Could you check a few things on this model? Use its own coordinates, in mm. Give positions to 0.01 mm unless a question says otherwise; leave off trailing zeros. Order: outer loops, then holes, each group sorted by start corner. A loop starts at its lowest first (then second) coordinate and runs counter-clockwise, first axis right, second up.
Autodesk Inventor part; units mm, degrees
ref_plane "YZ Plane" through (0, 0, 0) normal (1, 0, 0) x (0, 1, 0)
ref_plane "XZ Plane" through (0, 0, 0) normal (0, 1, 0) x (-1, 0, 0)
ref_plane "XY Plane" through (0, 0, 0) normal (0, 0, 1) x (1, 0, 0)
sketch "Sketch1" plane through (0, 0, 0) normal (1, 0, 0) x (0, 1, 0)
  line L0 (0, 78.3368) -> (0, 427.0775)
  line L1 (9.8481, 428.814) -> (120.1519, 448.2635)
  line L2 (131.7365, 440.1519) -> (154.2135, 312.6787)
  line L3 (503.1119, 189.3047) -> (590.8645, 150.2346)
  line L4 (595.9326, 137.0318) -> (559.5861, 55.3964)
  line L5 (494.9423, 192.942) -> (494.9423, 192.942)
  line L6 (442.0149, 172.9748) -> (165.6696, 297.928)
  arc A0 (442.0149, 172.9748) -> (490.9347, 186.0198) centre (458.495, 209.4221) ccw
  arc A1 (154.2135, 312.6787) -> (165.6696, 297.928) centre (173.9096, 316.1516) ccw
  arc A2 (131.7365, 440.1519) -> (120.1519, 448.2635) centre (121.8884, 438.4154) ccw
  line L7 (9.8481, 428.814) -> (0, 417.0775)
  arc A3 (595.9326, 137.0318) -> (590.8645, 150.2346) centre (586.7972, 141.0991) ccw
  arc A4 (503.1119, 189.3047) -> (490.9347, 186.0198) centre (499.0446, 180.1692) ccw
  line L8 (9.651, 68.3429) -> (550.1017, 49.4699)
  arc A5 (550.1017, 49.4699) -> (559.5861, 55.3964) centre (550.4507, 59.4638) ccw
  arc A6 (0, 78.3368) -> (9.651, 68.3429) centre (10, 78.3368) ccw
  line L9 (0, 417.0775) -> (0, 78.3368)
  point P0 (534.922, 0)
  point P1 (130, 450)
  point P2 (156.0472, 302.2788)
  point P3 (600, 146.1672)
  point P4 (478.4622, 156.4947)
  point P5 (0, 427.0775)
  point P6 (0, 28.3368)
  dimension "d0" = 130
  dimension "d1" = 404.922
  dimension "d3" = 150
  dimension "d4" = 160
  dimension "d5" = 115
  dimension "d13" = 40
  dimension "d14" = 40
  dimension "d15" = 20
  dimension "d16" = 10
  dimension "d17" = 10
  dimension "d18" = 10
  dimension "d68" = 10
  dimension "d69" = 10
extrude "Extrusion1" add sketch "Sketch1" along normal blind 16
sketch "Sketch2" plane through (16, 0, 0) normal (1, 0, 0) x (0, 0, -1)
  line L0 (-172.9748, 442.0149) -> (-297.928, 165.6696)
  line L1 (-428.814, 9.8481) -> (-417.0775, 0)
  line L2 (-417.0775, 0) -> (-78.3368, 0)
  line L3 (-55.3964, 559.5861) -> (-137.0318, 595.9326)
  arc A0 (-137.0318, 595.9326) -> (-150.2346, 590.8645) centre (-141.0991, 586.7972) ccw
  line L4 (-150.2346, 590.8645) -> (-189.3047, 503.1119)
  arc A1 (-189.3047, 503.1119) -> (-186.0198, 490.9347) centre (-180.1692, 499.0446) ccw
  arc A2 (-172.9748, 442.0149) -> (-186.0198, 490.9347) centre (-209.4221, 458.495) ccw
  line L5 (-172.9748, 442.0149) -> (-297.928, 165.6696)
  arc A3 (-312.6787, 154.2135) -> (-297.928, 165.6696) centre (-316.1516, 173.9096) ccw
  line L6 (-312.6787, 154.2135) -> (-440.1519, 131.7365)
  arc A4 (-440.1519, 131.7365) -> (-448.2635, 120.1519) centre (-438.4154, 121.8884) ccw
  line L7 (-448.2635, 120.1519) -> (-428.814, 9.8481)
  line L8 (-438.4154, 121.8884) -> (-310.9422, 144.3654)
  line L9 (-286.9073, 160.6932) -> (-163.5511, 437.7551)
  line L10 (-163.5511, 437.7551) -> (-143.4328, 482.9414)
  line L11 (-143.4328, 482.9414) -> (-139.4594, 491.8657)
  line L12 (-139.4594, 491.8657) -> (-130.324, 487.7983)
  line L13 (-130.324, 487.7983) -> (-288.9516, 131.5158)
  line L14 (-288.9516, 131.5158) -> (-298.087, 135.5831)
  line L15 (-298.087, 135.5831) -> (-286.9073, 160.6932)
  line L16 (-428.814, 9.8481) -> (-417.0775, 0)
  line L17 (-143.5969, 482.7615) -> (-143.5268, 482.7303)
  line L18 (-438.4154, 121.8884) -> (-303.4968, 145.6782)
  line L19 (-303.4968, 145.6782) -> (-301.7603, 135.8301)
  line L20 (-301.7603, 135.8301) -> (-436.679, 112.0403)
  line L21 (-438.4154, 121.8884) -> (-436.679, 112.0403)
  line L22 (-436.679, 112.0403) -> (-417.404, 2.7267)
  line L23 (-436.679, 112.0403) -> (-325.679, 112.0403) construction
  line L24 (-417.404, 2.7267) -> (-407.5559, 4.4631)
  line L25 (-407.5559, 4.4631) -> (-426.8309, 113.7768)
  line L26 (-141.0991, 586.7972) -> (-182.9931, 492.702)
  line L27 (-182.9931, 492.702) -> (-173.8576, 488.6347)
  line L28 (-173.8576, 488.6347) -> (-131.9637, 582.7298)
  line L29 (-139.4594, 491.8657) -> (-166.9664, 504.1126)
  line L30 (-139.4594, 491.8657) -> (-109.3492, 491.8657) construction
  line L31 (-166.9664, 504.1126) -> (-171.0338, 494.9772)
  line L32 (-171.0338, 494.9772) -> (-143.5268, 482.7303)
  line L33 (-141.0991, 586.7972) -> (-131.9637, 582.7298)
  line L34 (-131.9637, 582.7298) -> (3.0363, 582.7298) construction
  line L35 (-12.7024, 518.6849) -> (487.2976, 518.6849) construction
  line L36 (-288.9516, 131.5158) -> (-274.7158, 163.4898)
  line L37 (-274.7158, 163.4898) -> (-214.4218, 136.6452)
  line L38 (-214.4218, 136.6452) -> (-218.4892, 127.5097)
  line L39 (-218.4892, 127.5097) -> (-278.7831, 154.3544)
  line L40 (-68.3429, 9.651) -> (-49.4699, 550.1017)
  arc A5 (-49.4699, 550.1017) -> (-55.3964, 559.5861) centre (-59.4638, 550.4507) ccw
  arc A6 (-78.3368, 0) -> (-68.3429, 9.651) centre (-78.3368, 10) ccw
  line L41 (-131.9637, 582.7298) -> (-54.3123, 548.1572)
  line L42 (-131.9637, 582.7298) -> (-46.9637, 582.7298) construction
  line L43 (-54.3123, 548.1572) -> (-58.3797, 539.0217)
  line L44 (-136.0311, 573.5943) -> (-58.3797, 539.0217)
  line L45 (-170.9977, 396.4438) -> (-86.038, 358.6172)
  line L46 (-86.038, 358.6172) -> (-155.1834, 203.3146)
  line L47 (-155.1834, 203.3146) -> (-146.0479, 199.2472)
  line L48 (-146.0479, 199.2472) -> (-76.9026, 354.5499)
  line L49 (-76.9026, 354.5499) -> (-86.038, 358.6172)
  point P0 (0, 0)
  dimension "d25" = 10
  dimension "d26" = 390
  dimension "d27" = 10
  dimension "d37" = 137
  dimension "d38" = 111
  dimension "d39" = 80
  dimension "d40" = 10
  dimension "d41" = 90
  dimension "d42" = 90
  dimension "d43" = 103
  dimension "d44" = 10
  dimension "d45" = 90
  dimension "d46" = 156
  dimension "d60" = 35
  dimension "d61" = 66
  dimension "d62" = 90
  dimension "d63" = 10
  dimension "d64" = 90
  dimension "d65" = 90
  dimension "d70" = 85
  dimension "d71" = 24
  dimension "d72" = 93
  dimension "d73" = 100
  dimension "d74" = 170
  dimension "d75" = 10
extrude "Extrusion2" cut sketch "Sketch2" against normal blind 7 contours L8 L18 L19 L20 L21 | L20 L25 L24 L22 | L49 L48 L47 L46 | L9 L10 L11 L12 L13 L14 L15 | L17 L32 L28 L29 L11 L10 | L13 L37 L38 L39 | L28 L27 L26 L33 | L28 L41 L43 L44
properties part number "Arcade_Left"
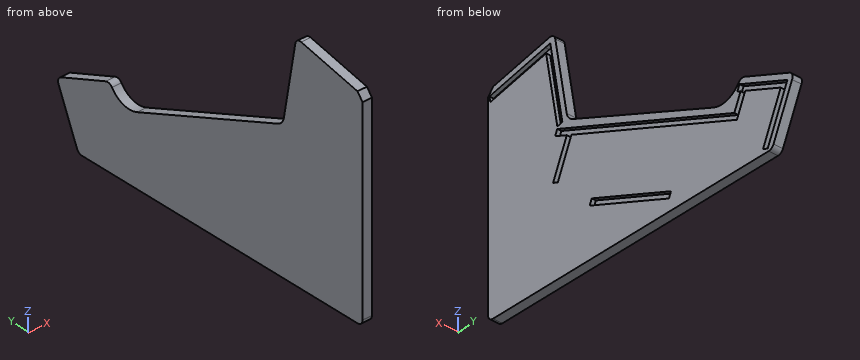
Item 1: Imagine slicing it at C-C on y = 449.5. List the corners of the cut face in (x, z) for me.
Findings:
outline: (0, 52.98) - (16, 52.98) - (16, 147.38) - (9, 147.38) - (9, 158.32) - (16, 158.32) - (16, 170.45) - (0, 170.45) - close
Item 2: For pin 1 (1 mm diameter, centred on x = 9, y = 406.5, fed in from -Z); pin 2 (5 mm diameter, centred on x = 7.5, y = 96.5, fed in from +Z); pin 3 (3 mm diameter, centred on y = 519.5, z = 174, fed in from -X); pin 4 (8 mm diameter, centred on x = 6.5, y = 261.5, fed in from +Z), each with a flat end and sliding along its axis, tell me the tip position at first contact or that it passes through.
Findings:
pin 1: stops at z = 54.47
pin 2: stops at z = 444.53
pin 3: stops at x = 0
pin 4: stops at z = 256.41
Item 3: Please list where these lines run through material, in increasing order: line 1 along Z through (x, y) = (12, 345); line 2 along Y through (x, z) = (5.75, 311.5); line 3 along Z through (x, y) = (14.5, 542).
Findings:
line 1: z = 56.63 to 81.15, 92.1 to 193.9, 204.85 to 216.84
line 2: y = 0 to 154.46
line 3: z = 49.75 to 57.05, 65.07 to 150.1, 161.04 to 171.99
Item 4: Imagine slicing it at B-B on z = 391. List the corners of the cut face in (x, y) for me, then the cut area to 3 significant figures.
Findings:
outline: (0, 0) - (16, 0) - (16, 120.09) - (9, 120.09) - (9, 130.25) - (16, 130.25) - (16, 140.4) - (0, 140.4) - close
area: 2,180 mm2
Item 5: Imagine slicing it at A-A on x = 4. List the corners of the cut face in (y, z) for me (1 decimal), then the cut area to 3 significant figures.
Findings:
outline: (0, 78.3) arc R10 ccw to (9.7, 68.3) - (550.1, 49.5) arc R10 ccw to (559.6, 55.4) - (595.9, 137) arc R10 ccw to (590.9, 150.2) - (503.1, 189.3) arc R10 ccw to (490.9, 186) arc R40 cw to (442, 173) - (165.7, 297.9) arc R20 cw to (154.2, 312.7) - (131.7, 440.2) arc R10 ccw to (120.2, 448.3) - (9.8, 428.8) - (0, 417.1) - close
area: 125,000 mm2
Item 6: Imagine slicing it at D-D on z = 238. List the corners of the cut face in (x, y) for me, then the cut area to 3 significant figures.
Findings:
outline: (0, 0) - (16, 0) - (16, 136.2) - (9, 136.2) - (9, 147.14) - (16, 147.14) - (16, 245.95) - (9, 245.95) - (9, 270.54) - (16, 270.54) - (16, 298.21) - (0, 298.21) - close
area: 4,520 mm2
